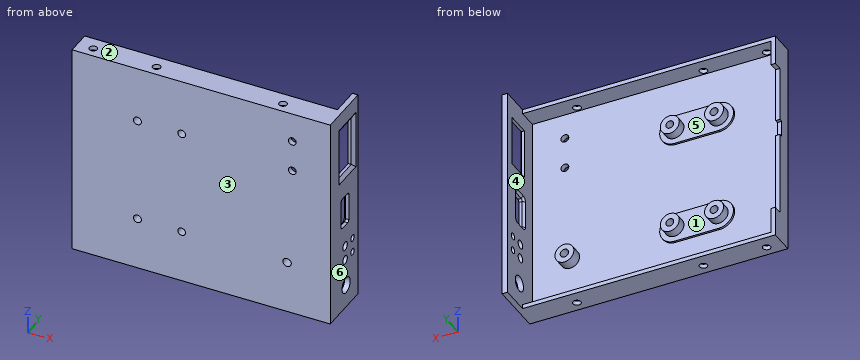
```python
from build123d import *

# Parameters (mm, degrees)
SKETCH_1_W             = 122.5
SKETCH_1_H             = 101.6
EXTRUDE_1_DEPTH        = 25.4
SKETCH_2_W             = 117.9
SKETCH_2_H             = 97.6
CUT_EXTRUDE_1_DEPTH    = 22.857
CUT_EXTRUDE_2_REACH    = 133.758
SKETCH_5_W             = 119.9
SKETCH_5_H             = 13.8
CUT_EXTRUDE_3_REACH    = 142.716
SKETCH_6_W             = 73.5
SKETCH_6_H             = 4.25
CUT_EXTRUDE_4_REACH    = 142.716
SKETCH_7_W             = 7.65
SKETCH_7_H             = 1.6
CUT_EXTRUDE_5_REACH    = 133.758
SKETCH_8_R             = 1.85
EXTRUDE_2_DEPTH        = 1
SKETCH_11_R            = 4.5
EXTRUDE_3_DEPTH        = 4.3
CUT_EXTRUDE_6_REACH    = 106.165
SKETCH_13_R            = 1.85
SKETCH_14_R            = 4.5
SKETCH_14_R_2          = 2
EXTRUDE_5_DEPTH        = 5.3
SKETCH_15_R            = 1.55
SKETCH_15_R_2          = 2.05
CUT_EXTRUDE_7_DEPTH    = 5.3
SKETCH_16_W            = 15
SKETCH_16_H            = 7
CUT_EXTRUDE_8_DEPTH    = 5.3
FILLET_1_R             = 1
SKETCH_17_W            = 23.7
SKETCH_17_H            = 11.5
CUT_EXTRUDE_9_DEPTH    = 5.3
CHAMFER_2_SIZE         = 2
CHAMFER_2_SIZE2        = 1.154700538
SKETCH_12_R            = 1.9
CUT_EXTRUDE_10_DEPTH   = 7.843
CUT_EXTRUDE_START      = -2.543
SKETCH_18_R            = 2
CUT_EXTRUDE_11_DEPTH   = 2.543
SKETCH_19_R            = 3.75
CUT_EXTRUDE_12_DEPTH   = 10
PATTERN_LINEAR_1_COUNT = 2
PATTERN_LINEAR_1_PITCH = 50
SKETCH_30_R            = 1.85
CUT_EXTRUDE_17_DEPTH   = 10
CHAMFER_3_SIZE         = 1


with BuildPart() as part:
    # Sketch 1 → Extrude 1 (new body)
    with BuildSketch(Plane(origin=(0, 0, 0), x_dir=(1, 0, 0), z_dir=(0, 1, 0))):
        with Locations((-18.703264605, -13.616494845)):
            Rectangle(SKETCH_1_W, SKETCH_1_H)
    extrude(amount=EXTRUDE_1_DEPTH)

    # Sketch 2 → Cut-Extrude 1 (cut)
    with BuildSketch(Plane(origin=(0, 25.4, 0), x_dir=(1, 0, 0), z_dir=(0, 1, 0))):
        with Locations((-19.003264605, -13.616494845)):
            Rectangle(SKETCH_2_W, SKETCH_2_H)
    extrude(amount=-CUT_EXTRUDE_1_DEPTH, mode=Mode.SUBTRACT)

    # Sketch 5 → Cut-Extrude 2 (cut, up to next)
    with BuildSketch(Plane(origin=(0, 0, -37.183505155), x_dir=(-1, 0, 0), z_dir=(0, 0, -1)), mode=Mode.PRIVATE) as cut_extrude_2_sk1:
        with Locations((20.003264605, 18.5)):
            Rectangle(SKETCH_5_W, SKETCH_5_H)
    cut_extrude_2_tool1 = extrude(cut_extrude_2_sk1.sketch, amount=-CUT_EXTRUDE_2_REACH, mode=Mode.PRIVATE) & part.part
    add(cut_extrude_2_tool1.solids().sort_by_distance((-20.003265, 18.5, -37.183505))[0], mode=Mode.SUBTRACT)

    # Sketch 6 → Cut-Extrude 3 (cut, up to next)
    with BuildSketch(Plane.ZY.offset(79.953264605), mode=Mode.PRIVATE) as cut_extrude_3_sk1:
        with Locations((13.666494845, 9.475)):
            Rectangle(SKETCH_6_W, SKETCH_6_H)
    cut_extrude_3_tool1 = extrude(cut_extrude_3_sk1.sketch, amount=-CUT_EXTRUDE_3_REACH, mode=Mode.PRIVATE) & part.part
    add(cut_extrude_3_tool1.solids().sort_by_distance((-79.953265, 9.475, 13.666495))[0], mode=Mode.SUBTRACT)

    # Sketch 7 → Cut-Extrude 4 (cut, up to next)
    with BuildSketch(Plane.ZY.offset(79.953264605), mode=Mode.PRIVATE) as cut_extrude_4_sk1:
        with Locations((20.591494845, 6.55)):
            Rectangle(SKETCH_7_W, SKETCH_7_H)
    cut_extrude_4_tool1 = extrude(cut_extrude_4_sk1.sketch, amount=-CUT_EXTRUDE_4_REACH, mode=Mode.PRIVATE) & part.part
    add(cut_extrude_4_tool1.solids().sort_by_distance((-79.953265, 6.55, 20.591495))[0], mode=Mode.SUBTRACT)

    # Sketch 8 → Cut-Extrude 5 (cut, up to next)
    with BuildSketch(Plane.XY.offset(64.416494845), mode=Mode.PRIVATE) as cut_extrude_5_sk1:
        with Locations((17.546735395, 5)):
            Circle(SKETCH_8_R)
    cut_extrude_5_tool1 = extrude(cut_extrude_5_sk1.sketch, amount=-CUT_EXTRUDE_5_REACH, mode=Mode.PRIVATE) & part.part
    # Sketch 8 → Cut-Extrude 5 (cut, up to next)
    with BuildSketch(Plane.XY.offset(64.416494845), mode=Mode.PRIVATE) as cut_extrude_5_sk2:
        with Locations((-42.453264605, 5)):
            Circle(SKETCH_8_R)
    cut_extrude_5_tool2 = extrude(cut_extrude_5_sk2.sketch, amount=-CUT_EXTRUDE_5_REACH, mode=Mode.PRIVATE) & part.part
    # Sketch 8 → Cut-Extrude 5 (cut, up to next)
    with BuildSketch(Plane.XY.offset(64.416494845), mode=Mode.PRIVATE) as cut_extrude_5_sk3:
        with Locations((-72.453264605, 5)):
            Circle(SKETCH_8_R)
    cut_extrude_5_tool3 = extrude(cut_extrude_5_sk3.sketch, amount=-CUT_EXTRUDE_5_REACH, mode=Mode.PRIVATE) & part.part
    cut_extrude_5_1 = cut_extrude_5_tool1.solids().sort_by_distance((17.546735, 5, 64.416495))[0]
    add(cut_extrude_5_1, mode=Mode.SUBTRACT)
    cut_extrude_5_2 = cut_extrude_5_tool2.solids().sort_by_distance((-42.453265, 5, 64.416495))[0]
    add(cut_extrude_5_2, mode=Mode.SUBTRACT)
    cut_extrude_5_3 = cut_extrude_5_tool3.solids().sort_by_distance((-72.453265, 5, 64.416495))[0]
    add(cut_extrude_5_3, mode=Mode.SUBTRACT)
    cut_extrude_5 = cut_extrude_5_1 + cut_extrude_5_2 + cut_extrude_5_3  # Cut-Extrude 5 as one shape, for the pattern or mirror that repeats it

    # Mirror 1: Cut-Extrude 5 across plane
    add(cut_extrude_5.mirror(Plane.XY.offset(13.616494845)), mode=Mode.SUBTRACT)

    # Sketch 10 → Extrude 2 (add)
    with BuildSketch(Plane(origin=(0, 2.543, 0), x_dir=(1, 0, 0), z_dir=(0, 1, 0))):
        with BuildLine():
            Line((-48.953264605, 19.183505155), (-27.953264605, 19.183505155))
            ThreePointArc((-27.953264605, 19.183505155), (-20.953264605, 12.183505155), (-27.953264605, 5.183505155))
            Line((-27.953264605, 5.183505155), (-48.953264605, 5.183505155))
            ThreePointArc((-48.953264605, 5.183505155), (-55.953264605, 12.183505155), (-48.953264605, 19.183505155))
        make_face()
    extrude_2 = extrude(amount=EXTRUDE_2_DEPTH)

    # Sketch 11 → Extrude 3 (add)
    with BuildSketch(Plane(origin=(0, 3.543, 0), x_dir=(1, 0, 0), z_dir=(0, 1, 0))):
        with Locations(Location((-48.953264605, 12.183505155, 0), (0, 0, 90))):
            Circle(SKETCH_11_R)
        with Locations(Location((-27.953264605, 12.183505155, 0), (0, 0, 90))):
            Circle(SKETCH_11_R)
    extrude_3 = extrude(amount=EXTRUDE_3_DEPTH)

    # Sketch 13 → Cut-Extrude 6 (cut, up to next)
    with BuildSketch(Plane(origin=(0, 7.843, 0), x_dir=(1, 0, 0), z_dir=(0, 1, 0)), mode=Mode.PRIVATE) as cut_extrude_6_sk1:
        with Locations(Location((-27.953264605, 12.183505155, 0), (0, 0, 270))):
            Circle(SKETCH_13_R)
    cut_extrude_6_tool1 = extrude(cut_extrude_6_sk1.sketch, amount=-CUT_EXTRUDE_6_REACH, mode=Mode.PRIVATE) & part.part
    cut_extrude_6 = cut_extrude_6_tool1.solids().sort_by_distance((-27.953265, 7.843, -12.183505))[0]
    add(cut_extrude_6, mode=Mode.SUBTRACT)

    # Sketch 14 → Extrude 5 (add)
    with BuildSketch(Plane(origin=(0, 2.543, 0), x_dir=(1, 0, 0), z_dir=(0, 1, 0))):
        with Locations(Location((22.046735395, 12.183505155, 0), (0, 0, 270))):
            Circle(SKETCH_14_R)
        with Locations(Location((22.046735395, 12.183505155, 0), (0, 0, 270))):
            Circle(SKETCH_14_R_2, mode=Mode.SUBTRACT)
    extrude(amount=EXTRUDE_5_DEPTH)

    # Sketch 15 → Cut-Extrude 7 (cut)
    with BuildSketch(Plane(origin=(42.546735395, 0, 0), x_dir=(0, 0, -1), z_dir=(1, 0, 0))):
        with Locations((12.683505155, 20.4)):
            Circle(SKETCH_15_R)
        with Locations((12.683505155, 13.6)):
            Circle(SKETCH_15_R_2)
        with Locations((5.683505155, 20.4)):
            Circle(SKETCH_15_R)
        with Locations((5.683505155, 13.6)):
            Circle(SKETCH_15_R_2)
    extrude(amount=-CUT_EXTRUDE_7_DEPTH, mode=Mode.SUBTRACT)

    # Sketch 16 → Cut-Extrude 8 (cut)
    with BuildSketch(Plane(origin=(42.546735395, 0, 0), x_dir=(0, 0, -1), z_dir=(1, 0, 0))):
        with Locations((-12.316494845, 13.5)):
            Rectangle(SKETCH_16_W, SKETCH_16_H)
    extrude(amount=-CUT_EXTRUDE_8_DEPTH, mode=Mode.SUBTRACT)

    # Fillet 1
    fillet_1_edges = [part.edges().sort_by_distance(p)[0] for p in [
        (41.246735395, 10, 19.816494845),
        (41.246735395, 17, 19.816494845),
        (41.246735395, 17, 4.816494845),
        (41.246735395, 10, 4.816494845),
    ]]
    fillet(fillet_1_edges, radius=FILLET_1_R)

    # Sketch 17 → Cut-Extrude 9 (cut)
    with BuildSketch(Plane(origin=(42.546735395, 0, 0), x_dir=(0, 0, -1), z_dir=(1, 0, 0))):
        with Locations((-42.766494845, 15.75)):
            Rectangle(SKETCH_17_W, SKETCH_17_H)
    extrude(amount=-CUT_EXTRUDE_9_DEPTH, mode=Mode.SUBTRACT)

    # Chamfer 2
    chamfer_2_edges = [part.edges().sort_by_distance(p)[0] for p in [
        (42.546735395, 15.75, 54.616494845),
        (42.546735395, 10, 42.766494845),
        (42.546735395, 15.75, 30.916494845),
        (42.546735395, 21.5, 42.766494845),
    ]]
    chamfer_2_side = [part.faces().sort_by_distance(p)[0] for p in [
        (42.546735395, 12.7, -36.136236326),
    ]]
    chamfer(chamfer_2_edges, length=CHAMFER_2_SIZE, length2=CHAMFER_2_SIZE2, reference=chamfer_2_side[0])

    # Sketch 12 → Cut-Extrude 10 (cut)
    with BuildSketch(Plane(origin=(0, 7.843, 0), x_dir=(1, 0, 0), z_dir=(0, 1, 0))):
        with Locations(Location((-48.953264605, 12.183505155, 0), (0, 0, 270))):
            Circle(SKETCH_12_R)
    cut_extrude_10 = extrude(amount=-CUT_EXTRUDE_10_DEPTH, mode=Mode.SUBTRACT)

    # Sketch 18 → Cut-Extrude 11 (cut)
    with BuildSketch(Plane(origin=(0, 2.543, 0), x_dir=(1, 0, 0), z_dir=(0, 1, 0)).offset(CUT_EXTRUDE_START)):
        with Locations(Location((22.046735395, 12.183505155, 0), (0, 0, 270))):
            Circle(SKETCH_18_R)
    extrude(amount=CUT_EXTRUDE_11_DEPTH, mode=Mode.SUBTRACT)

    # Sketch 19 → Cut-Extrude 12 (cut)
    with BuildSketch(Plane.ZY.offset(-39.946735395)):
        with Locations((-26.183505155, 14.543)):
            Circle(SKETCH_19_R)
    extrude(amount=-CUT_EXTRUDE_12_DEPTH, mode=Mode.SUBTRACT)

    # Pattern Linear 1: Extrude 2, Extrude 3, Cut-Extrude 6, Cut-Extrude 10 ×2
    with Locations(*[(0, 0, i * PATTERN_LINEAR_1_PITCH) for i in range(1, PATTERN_LINEAR_1_COUNT)]):
        add(extrude_2)
        add(extrude_3)
        add(cut_extrude_6, mode=Mode.SUBTRACT)
        add(cut_extrude_10, mode=Mode.SUBTRACT)

    # Sketch 30 → Cut-Extrude 17 (cut)
    with BuildSketch(Plane(origin=(0, 2.543, 0), x_dir=(1, 0, 0), z_dir=(0, 1, 0))):
        with Locations(Location((24.546735395, -50.416494845, 0), (0, 0, 270))):
            Circle(SKETCH_30_R)
        with Locations(Location((24.546735395, -35.416494845, 0), (0, 0, 270))):
            Circle(SKETCH_30_R)
    extrude(amount=-CUT_EXTRUDE_17_DEPTH, mode=Mode.SUBTRACT)

    # Chamfer 3
    chamfer_3_edges = [part.edges().sort_by_distance(p)[0] for p in [
        (39.946735395, 13.5, 4.816494845),
        (39.946735395, 10, 12.316494845),
        (39.946735395, 13.5, 19.816494845),
        (39.946735395, 17, 12.316494845),
        (39.946735395, 10.292893219, 5.109388064),
        (39.946735395, 10.292893219, 19.523601627),
        (39.946735395, 16.707106781, 5.109388064),
        (39.946735395, 16.707106781, 19.523601627),
    ]]
    chamfer(chamfer_3_edges, length=CHAMFER_3_SIZE)


solid = part.part
```
Here's how the part is built. I have some questions about the finished solid (model axes, mm). Face numbers are marked on the shaded views. A direction names the side the tool comes from. Give positions to 0.01 mm unless a question says otherwise; leave off trailing zeros. Order: outer loops, then holes, each group sorted by start corner. A loop starts at its lowest first (then second) coordinate and runs counter-clockwise, first axis right, second up. Notation, with made-up numbers: (48, 24) -> (72, 24) arc R20 ccw to (72, 40) -> close; hole circle Ø1 at (45, 0.25). An arc over 180 degrees is marked (long way). Use CSV: the item, a comma, the result in double quotes. Start each with the question number.
Item 1: If I drill on probe 1 along Z at (x, y) = (-45.5, 11.5); probe 2 along Z at (x, y) = (23, 4.5); probe 3 along X at (y, z) = (7.25, 60.5), over which ranges is the centre line in solid material (lowest first)? Write a range as [from, to].
Item 2: Suppose I cut it at A-A (x = -37). List the corners of the cut face in (y, z) for me.
Item 3: I'm going to push flat-ended pins straight in: P1, Ø4.5, axis at y = 13.6, z = -5.68, coming from the -X side; P2, Ø4.5, axis at x = -48.5, z = -10, coming from the +Y side; P3, Ø4, axis at x = -43, z = 35, coming from the +Y side. Where does each tip first touch, or does it pass through?
Item 4: Thinking about a two-plate mould opening in X: for the marked faces 3, 4, 5 and 6, which applies, pulls with the +X half, pulls with the -X half, needs draft (parallel to the pull), parting line crosses it, or undercut?
Item 5: On a 3-axis mill with a long thin cutter (end or side, diameter ignored), from which of +Z, -Z, +X, -X, +Y, -Y can I reach the whole of each face in a straight line? I mean the marked faces 1 and 2. Say none if no direction works.
Answer block:
1,probe 1,"z = [-37.18, -35.18], [62.42, 64.42]"
1,probe 2,"z = [-37.18, -35.18], [-16.58, -13.94], [-10.43, -7.79], [62.42, 64.42]"
1,probe 3,"x = [-79.95, -77.95], [39.95, 42.55]"
2,outline,"(0, -37.18) -> (11.6, -37.18) -> (11.6, -35.18) -> (2.54, -35.18) -> (2.54, -19.18) -> (3.54, -19.18) -> (3.54, -5.18) -> (2.54, -5.18) -> (2.54, 30.82) -> (3.54, 30.82) -> (3.54, 44.82) -> (2.54, 44.82) -> (2.54, 62.42) -> (11.6, 62.42) -> (11.6, 64.42) -> (0, 64.42) -> close"
3,P1,"stops at x = 39.95"
3,P2,"stops at y = 7.84"
3,P3,"stops at y = 3.54"
4,face 3,"needs draft"
4,face 4,"undercut"
4,face 5,"undercut"
4,face 6,"pulls with the +X half"
5,face 1,"+Y"
5,face 2,"+Z, +X, -X, +Y, -Y"
